```python
from build123d import *

# Parameters (mm, degrees)
BOSS_EXTRUDE1_DEPTH = 8
SKETCH5_R           = 2.1
CUT_EXTRUDE1_DEPTH  = 5
SKETCH6_R           = 1.65
CUT_EXTRUDE2_DEPTH  = 36
FILLET1_R           = 2


with BuildPart() as part:
    # Sketch3 → Boss-Extrude1 (new body)
    with BuildSketch(Plane.XY):
        with BuildLine():
            Line((-31.937438845, -2), (-45.623026261, -2))
            Line((-45.623026261, -2), (-45.623026261, -10))
            Line((-45.623026261, -10), (-35.623026261, -10))
            ThreePointArc((-35.623026261, -10), (0, -37), (35.623026261, -10))
            Line((35.623026261, -10), (45.623026261, -10))
            Line((45.623026261, -10), (45.623026261, -2))
            Line((45.623026261, -2), (31.937438845, -2))
            ThreePointArc((31.937438845, -2), (0, -32), (-31.937438845, -2))
        make_face()
    extrude(amount=BOSS_EXTRUDE1_DEPTH)

    # Sketch5 → Cut-Extrude1 (cut)
    with BuildSketch(Plane.XZ.offset(2)):
        with Locations((40.623026261, 4)):
            Circle(SKETCH5_R)
    cut_extrude1 = extrude(amount=CUT_EXTRUDE1_DEPTH, mode=Mode.SUBTRACT)

    # Sketch6 → Cut-Extrude2 (cut, through all)
    with BuildSketch(Plane(origin=(0, -2, 0), x_dir=(1, 0, 0), z_dir=(0, 1, 0))):
        with Locations((40.623026261, -4)):
            Circle(SKETCH6_R)
    cut_extrude2 = extrude(amount=-CUT_EXTRUDE2_DEPTH, mode=Mode.SUBTRACT)

    # Mirror1: Cut-Extrude1, Cut-Extrude2 across plane
    add(cut_extrude1.mirror(Plane(origin=(0, 0, 0), x_dir=(0, 0, 1), z_dir=(1, 0, 0))), mode=Mode.SUBTRACT)
    add(cut_extrude2.mirror(Plane(origin=(0, 0, 0), x_dir=(0, 0, 1), z_dir=(1, 0, 0))), mode=Mode.SUBTRACT)

    # Fillet1
    fillet1_edges = [part.edges().sort_by_distance(p)[0] for p in [
        (-45.623026261, -2, 4),
        (-31.937438845, -2, 4),
        (31.937438845, -2, 4),
        (45.623026261, -2, 4),
        (45.623026261, -10, 4),
        (35.623026261, -10, 4),
        (-35.623026261, -10, 4),
        (-45.623026261, -10, 4),
    ]]
    fillet(fillet1_edges, radius=FILLET1_R)


solid = part.part
```
CAD build for the part. Positions are in the model's coordinates, mm. A direction names the side the tool comes from. Round coordinates to 2 decimals unless told otherwise and drop trailing zeros. Order: outer loops, then holes, each group sorted by start corner. A loop starts at its lowest first (then second) coordinate and runs counter-clockwise, first axis right, second up.
Item 1: Saw through at C-C on y = -17.5. Write the cut outline in (x, z), then the cut area to 3 significant figures.
Item 2: Saw through at B-B on y = -5.5. Write the cut outline in (x, z).
Item 3: Probe line 1 along X through (y, z) = (-14, 7); line 2 along X through (y, z) = (-26, 5.5); line 3 along Y through (x, z) = (1, 2.25). List the from-to ranges inside material, lowest first.
Item 4: Saw through at D-D on x = -9.5. Write the cut outline in (y, z).
Item 5: Mould opens along Z. For faces 5 (the face through (-38.525, -4.465, 4.092)), 6 (the face through (38.525, -4.465, 4.092)), 7 (the face through (-0.2, -32.4, 8)), 8 (the face through (45.02, -9.43, 4.06)) say: pulls with the +Z half, pulls with the -Z half, needs draft (parallel to the pull), parting line crosses it, or undercut.
Item 6: Saw through at A-A on z = 4. State how many separate pieces and enclosed holes the cut face has, then the cut area to 3 significant figures.
Item 7: Pin check, flat tips, straight feed: pin 1 (4.5 mm diameter, centred on x = 40, z = 4.5, fed in from +Y); pin 2 (1 mm diameter, centred on x = 5.5, z = 3.5, fed in from -Y); pin 3 (3.5 mm diameter, centred on x = -40.62, z = 4, fed in from -Y); pin 4 (1 mm diameter, centred on y = -9.5, z = 6, fed in from +X). Stop position of each tip, or through.
Item 8: Tool access for faces 1 (the face through (-32.45, -2.49, 4.06)), 2 (the face through (38, -2, 4)), 3 (the face through (-39, -7, 3)), 4 (the face through (39, -10, 5)): list every direction of +Z, -Z, +X, -X, +Y, -Y with a clear straight run to the whole face (end or side of a thin tool).
Reported:
1. outline: (-32.6, 0) - (-26.79, 0) - (-26.79, 8) - (-32.6, 8) - close; (26.79, 0) - (32.6, 0) - (32.6, 8) - (26.79, 8) - close
1. area: 92.9 mm2
2. outline: (-45.62, 0) - (-31.52, 0) - (-31.52, 8) - (-45.62, 8) - close; (31.52, 0) - (45.62, 0) - (45.62, 8) - (31.52, 8) - close; hole circle Ø4.2 at (-40.62, 4); hole circle Ø4.2 at (40.62, 4)
3. line 1: x = -34.25 to -28.77, 28.77 to 34.25
3. line 2: x = -26.32 to -18.65, 18.65 to 26.32
3. line 3: y = -36.99 to -31.98
4. outline: (-35.76, 0) - (-30.56, 0) - (-30.56, 8) - (-35.76, 8) - close
5. face 5: undercut
5. face 6: undercut
5. face 7: pulls with the +Z half
5. face 8: needs draft
6. separate pieces: 3
6. enclosed holes: 0
6. area: 603 mm2
7. pin 1: stops at y = -2
7. pin 2: stops at y = -36.66
7. pin 3: stops at y = -10
7. pin 4: stops at x = 45.36
8. face 1: +Z, -Z, +Y
8. face 2: +Z, -Z, +X, -X, +Y
8. face 3: +Y
8. face 4: +Z, -Z, +X, -Y
